Part model, mm, in its own coordinate system. Face numbers are marked on the shaded views. Coordinates: 2 decimals unless noted, no trailing zeros. Loops run counter-clockwise (first coordinate to the right, second up) from the corner with the lowest first, then second, coordinate; pieces in that order, holes last. Notation, with made-up numbers: M 17.25,68.5 L 43.25,68.5 A18 cw 43.25,93.5 Z; hole C -37,38 d11. An arc over 180 degrees is marked long. Use a Markdown table: item, result. Add a question column.
1) Pin check, flat tips, straight feed: pin 1 Ø1.5 at (y, z) = (8.5, 2) entering from +X; pin 2 Ø2 at (x, y) = (2, 5) entering from -Z. Stop position of each tip, or through.
2) Wall check: probe 1 along Z at (x, y) = (0, 0.05); probe 2 along Y at (x, z) = (-1.5, -0.5); probe 3 along Z at (x, y) = (0.1, 9). Give the ranges that are in metal, low to high. Write a range as from..to.
3) Band-saw the part on A-A (x = 0). List the corners of the cut face in (y, z), plus the area to 3 significant figures.
4) Band-saw the part on C-C (y = 10.75). List the corners of the cut face in (x, z), plus the area to 3 significant figures.
5) Pull direction X, two halves, no side cores. Call the marked faces 1 and 2: released by +X, released by -X, zero draft, split by the parting line, or undercut.
6) Band-saw the part on B-B (z = 0). List the corners of the cut face in (x, y), plus the area to 3 significant figures.
7) Band-saw the part on D-D (z = 2). List the corners of the cut face in (x, y), plus the area to 3 significant figures.
from build123d import *

# Parameters (mm, degrees)
SKETCH2_R           = 3
BOSS_EXTRUDE1_DEPTH = 12
SKETCH3_R           = 1
BOSS_EXTRUDE2_DEPTH = 0.3
SKETCH4_R           = 0.25
CUT_EXTRUDE1_DEPTH  = 0.1


with BuildPart() as part:
    # Sketch2 → Boss-Extrude1 (new body)
    with BuildSketch(Plane(origin=(0, 0, 0), x_dir=(1, 0, 0), z_dir=(0, 1, 0))):
        Circle(SKETCH2_R)
    extrude(amount=BOSS_EXTRUDE1_DEPTH)

    # Sketch3 → Boss-Extrude2 (add)
    with BuildSketch(Plane(origin=(0, 12, 0), x_dir=(1, 0, 0), z_dir=(0, 1, 0))):
        Circle(SKETCH3_R)
    extrude(amount=BOSS_EXTRUDE2_DEPTH)

    # Sketch4 → Cut-Extrude1 (cut)
    with BuildSketch(Plane(origin=(0, 0, 0), x_dir=(-1, 0, 0), z_dir=(0, -1, 0))):
        with Locations((0, 2)):
            Circle(SKETCH4_R)
        with Locations((0, -2)):
            Circle(SKETCH4_R)
    extrude(amount=-CUT_EXTRUDE1_DEPTH, mode=Mode.SUBTRACT)


solid = part.part
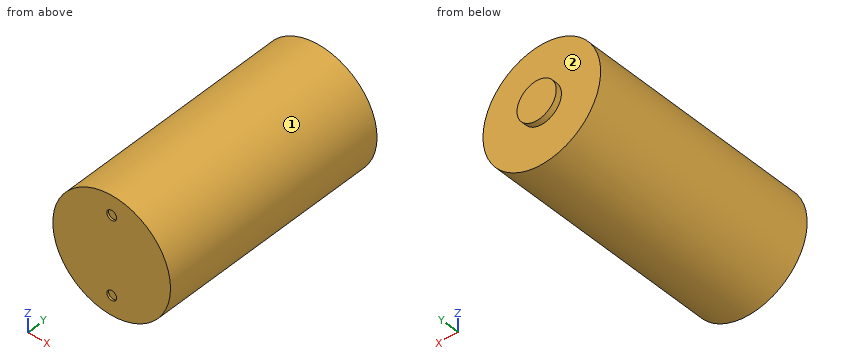
Entries:
| question | item | result |
|---|---|---|
| 1 | pin 1 | x = 2.73 |
| 1 | pin 2 | z = -2.83 |
| 2 | probe 1 | -3..-2.25, -1.75..1.75, 2.25..3 |
| 2 | probe 2 | 0..12 |
| 2 | probe 3 | -3..3 |
| 3 | outline | M 0,-3 L 12,-3 L 12,-1 L 12.3,-1 L 12.3,1 L 12,1 L 12,3 L 0,3 L 0,2.25 L 0.1,2.25 L 0.1,1.75 L 0,1.75 L 0,-1.75 L 0.1,-1.75 L 0.1,-2.25 L 0,-2.25 Z |
| 3 | area | 72.5 mm2 |
| 4 | outline | C 0,0 d6 |
| 4 | area | 28.3 mm2 |
| 5 | face 1 | split by the parting line |
| 5 | face 2 | zero draft |
| 6 | outline | M -3,0 L 3,0 L 3,12 L 1,12 L 1,12.3 L -1,12.3 L -1,12 L -3,12 Z |
| 6 | area | 72.6 mm2 |
| 7 | outline | M -2.24,0 L -0.25,0 L -0.25,0.1 L 0.25,0.1 L 0.25,0 L 2.24,0 L 2.24,12 L -2.24,12 Z |
| 7 | area | 53.6 mm2 |
